Geometry check sheet. Reference: the model listing, model coordinates, mm. Give positions to 0.01 mm unless a question says otherwise; leave off trailing zeros. Write each loop counter-clockwise with the first axis right and the second up, starting at its lowest first coordinate (ties: lowest second). Pieces come first, ordered by that corner, then holes. Notation, with made-up numbers: (-23.5, -17.75) -> (-18.5, -17.75) arc R14 cw to (-18.5, 0.25) -> close; hole circle Ø8 at (-2, 79.5). An arc over 180 degrees is marked (long way). One line per item, written item: value.
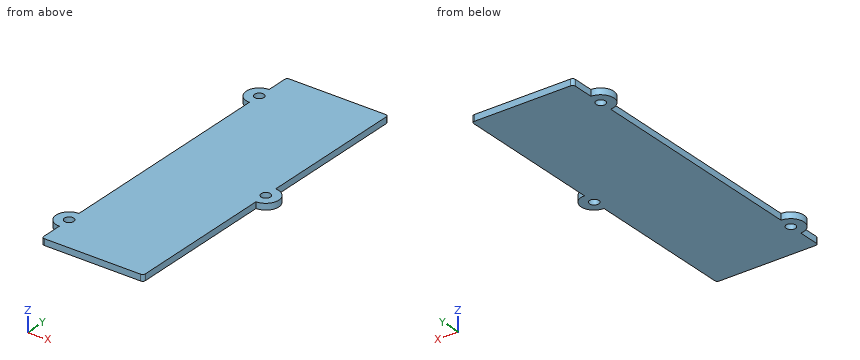
from build123d import *

# Parameters (mm, degrees)
SKETCH1_W           = 24.765
SKETCH1_H           = 79.375
BOSS_EXTRUDE1_DEPTH = 1.524
SKETCH2_R           = 3.175
BOSS_EXTRUDE2_DEPTH = 1.524
SKETCH3_R           = 1.143
CUT_EXTRUDE1_DEPTH  = 85.162680572
FILLET1_R           = 0.635


with BuildPart() as part:
    # Sketch1 → Boss-Extrude1 (new body)
    with BuildSketch(Plane.XY):
        with Locations((12.3825, 39.6875)):
            Rectangle(SKETCH1_W, SKETCH1_H)
    extrude(amount=BOSS_EXTRUDE1_DEPTH)

    # Sketch2 → Boss-Extrude2 (add)
    with BuildSketch(Plane.XY.offset(1.524)):
        with Locations((0, 8.89)):
            Circle(SKETCH2_R)
        with Locations((24.765, 39.6875)):
            Circle(SKETCH2_R)
        with Locations((0, 70.485)):
            Circle(SKETCH2_R)
    extrude(amount=-BOSS_EXTRUDE2_DEPTH)

    # Sketch3 → Cut-Extrude1 (cut, through all)
    with BuildSketch(Plane.XY.offset(1.524)):
        with Locations((0, 8.89)):
            Circle(SKETCH3_R)
        with Locations((24.765, 39.6875)):
            Circle(SKETCH3_R)
        with Locations((0, 70.485)):
            Circle(SKETCH3_R)
    extrude(amount=-CUT_EXTRUDE1_DEPTH, mode=Mode.SUBTRACT)

    # Fillet1
    fillet1_edges = [part.edges().sort_by_distance(p)[0] for p in [
        (0, 79.375, 0.762),
        (24.765, 79.375, 0.762),
        (24.765, 0, 0.762),
        (0, 0, 0.762),
    ]]
    fillet(fillet1_edges, radius=FILLET1_R)


solid = part.part
1) Sectioned sample at A-A on z = 0.65. Give the number of separate pieces and of enclosed holes in the cut face, plus the area to 3 significant figures.
Verdict:
separate pieces: 1
enclosed holes: 3
area: 2,000 mm^2
2) Sectioned sample at B-B on y = 55. Record the cut outline in (x, z) (3 decimals), plus the area to 3 significant figures.
Verdict:
outline: (0, 0) -> (24.765, 0) -> (24.765, 1.524) -> (0, 1.524) -> close
area: 37.7 mm^2
3) Depth check by flat-ended pin: pin 1 Ø0.5 at (y, z) = (42.5, 1) entering from -X; pin 2 Ø0.5 at (y, z) = (54, 0.5) entering from +X (3 decimals). Enter the tip coordinate at first touch or a pass-through.
Verdict:
pin 1: x = 0
pin 2: x = 24.765
4) Scan lines: probe 1 along Y at (x, z) = (0.5, 0.65); probe 2 along X at (y, z) = (29, 1.05) (3 decimals); probe 3 along Y at (x, z) = (-1, 1.2). Record each from-to range of solid material in increasing order.
Verdict:
probe 1: 0.01 to 7.86, 9.92 to 69.46, 71.51 to 79.36
probe 2: 0 to 24.765
probe 3: 5.88 to 8.34, 9.44 to 11.9, 67.47 to 69.93, 71.04 to 73.5
